Part print with two shaded views. Sizes in mm from the minimum x, y, z corner. A direction names the side the tool comes from. Round coordinates to 2 decimals unless told otherwise and drop trailing zeros. Write each loop counter-clockwise with the first axis right and the second up, starting at its lowest first coordinate (ties: lowest second). Pieces come first, ordered by that corner, then holes. Notation, with made-up numbers: (49, -34) -> (99, -34) arc R10 cw to (99, -20) -> close; hole circle Ø5 at (12.25, -10.75). An arc over 180 degrees is marked (long way). Return JSON: item names as keys, results as strings.
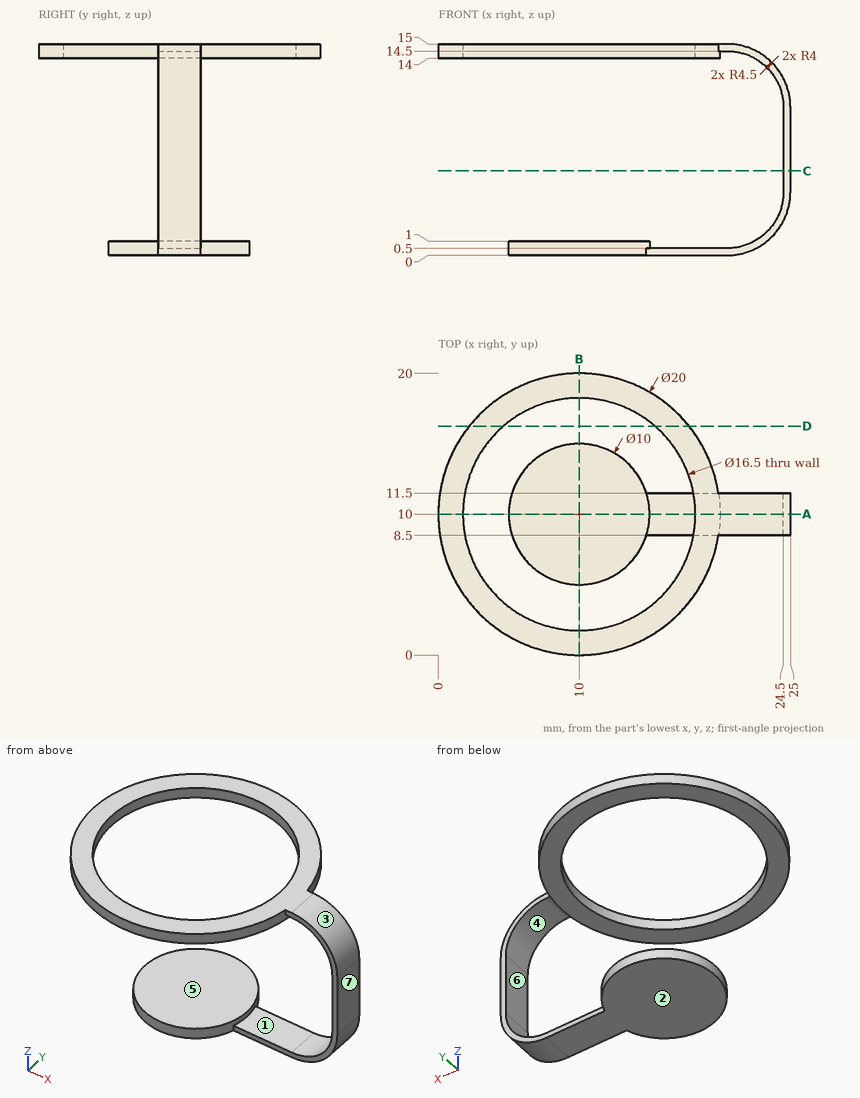
Q1. Wall check: L1, parallel to Y at x = 10, z = 14.8; L2, parallel to Z at x = 11.25, y = 1; L3, parallel to Z at x = 7.5, y = 9.5. Give the ranges that are in metal, low to high.
Verdict:
{"L1": "y = 0 to 1.75, 18.25 to 20", "L2": "z = 14 to 15", "L3": "z = 0 to 1"}
Q2. Saw through at A-A on y = 10. List the corners of the cut face in (x, z).
Verdict:
{"outline": "(0, 14) -> (1.75, 14) -> (1.75, 15) -> (0, 15) -> close; (5, 0) -> (20.5, 0) arc R4.5 ccw to (25, 4.5) -> (25, 10.5) arc R4.5 ccw to (20.5, 15) -> (18.25, 15) -> (18.25, 14) -> (20, 14) -> (20, 14.5) -> (20.5, 14.5) arc R4 cw to (24.5, 10.5) -> (24.5, 4.5) arc R4 cw to (20.5, 0.5) -> (15, 0.5) -> (15, 1) -> (5, 1) -> close"}
Q3. Two-plate mould, pull along Z, no slides. Class the marked faces 1, 2 and 3: +Z half, -Z half, draft (parallel to the pull), parting line (faces both ways), or undercut.
Verdict:
{"face 1": "undercut", "face 2": "-Z half", "face 3": "+Z half"}
Q4. 3-axis set-ups, long thin cutter, end or side, ignore diameter. For the marked faces 4, 5, 6 and 7: which of +Z, -Z, +X, -X, +Y, -Y reach the whole face in a straight line?
Verdict:
{"face 4": "+Y, -Y", "face 5": "+Z, -X, +Y, -Y", "face 6": "-X, +Y, -Y", "face 7": "+Z, -Z, +X, +Y, -Y"}
Q5. Saw through at B-B on x = 10. List the corners of the cut face in (y, z).
Verdict:
{"outline": "(0, 14) -> (1.75, 14) -> (1.75, 15) -> (0, 15) -> close; (5, 0) -> (15, 0) -> (15, 1) -> (5, 1) -> close; (18.25, 14) -> (20, 14) -> (20, 15) -> (18.25, 15) -> close"}
Q6. Saw through at C-C on z = 6. List the corners of the cut face in (x, y).
Verdict:
{"outline": "(24.5, 8.5) -> (25, 8.5) -> (25, 11.5) -> (24.5, 11.5) -> close"}
Q7. Pin check, flat tips, straight feed: pin 1 Ø3 at (x, y) = (9.5, 9.5) entering from +Z; pin 2 Ø1.5 at (y, z) = (10.5, 7.5) entering from -X. Stop position of each tip, or through.
Verdict:
{"pin 1": "stops at z = 1", "pin 2": "stops at x = 24.5"}
Q8. Saw through at D-D on y = 16.25. List the corners of the cut face in (x, z).
Verdict:
{"outline": "(2.19, 14) -> (4.61, 14) -> (4.61, 15) -> (2.19, 15) -> close; (15.39, 14) -> (17.81, 14) -> (17.81, 15) -> (15.39, 15) -> close"}
